Can you work these out from the model? Positions are in its coordinate system, mm. Face numbers are marked on the shaded views. A direction names the side the tool comes from. Give positions to 0.01 mm unless a question says otherwise; leave off trailing zeros. Loops run counter-clockwise (first coordinate to the right, second up) from the corner with the lowest first, then second, coordinate; pieces in that order, holes last. Notation, with made-up numbers: (80, 43) -> (86, 43) arc R25 ccw to (86, 60) -> close; hole circle Ø7 at (-19, 66). An arc over 180 degrees is marked (long way). One line per question, with ' | ' between items.
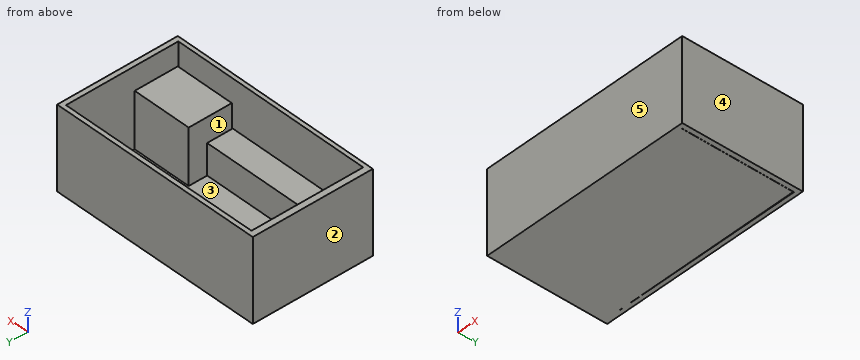
from build123d import *

# Parameters (mm, degrees)
F1_DEPTH = 76.708
F2_W     = 133.829683
F2_H     = 23.887876
F3_DEPTH = 32.512
F4_W     = 55.258706
F4_H     = 40.292808
F5_DEPTH = 55.372
F6_W     = 189.376198
F6_H     = 104.761295
F7_DEPTH = 3.81
F8_W     = 187.649362
F8_H     = 20.434209
F9_DEPTH = 35.306


with BuildPart() as f1:
    # F0 (on Top) → F1 (new body)
    with BuildSketch(Plane.XY):
        Polygon((99.436894, 56.841634), (-100.300305, 56.266025), (-100.300305, -55.97822), (99.436894, -55.97822), align=None)
        Polygon((-94.544195, -52.236743), (-94.544195, 52.236743), (94.832003, 52.81236), (94.832003, -52.236743), align=None, mode=Mode.SUBTRACT)
    extrude(amount=F1_DEPTH)

    # F2 (on Top) → F3 (join)
    with BuildSketch(Plane.XY):
        with Locations((-27.773253, -40.292805)):
            Rectangle(F2_W, F2_H)
    extrude(amount=F3_DEPTH)

    # F4 (on Top) → F5 (join)
    with BuildSketch(Plane.XY):
        with Locations((66.770941, -31.226925)):
            Rectangle(F4_W, F4_H)
    extrude(amount=F5_DEPTH)

    # F6 (on Top) → F7 (join)
    with BuildSketch(Plane.XY):
        with Locations((4e-06, -0.143905)):
            Rectangle(F6_W, F6_H)
    extrude(amount=F7_DEPTH)

    # F8 (on Top) → F9 (join)
    with BuildSketch(Plane.XY):
        with Locations((4e-06, 40.868416)):
            Rectangle(F8_W, F8_H)
    extrude(amount=F9_DEPTH)


solid = f1.part
Q1. For pin 1 Ø5 at (x, z) = (11.5, 43) entering from +Y; pin 2 Ø16.5 at (x, y) = (-46, 44.5) entering from +Z; pin 3 Ø25 at (x, z) = (41.5, 15.5) entering from +Y; pin 4 Ø20 at (x, y) = (64, -24) entering from +Z, each with a flat end and sliding along its axis, tell me the tip position at first contact or that it passes through.
Entries:
pin 1: y = 56.6 | pin 2: z = 76.71 | pin 3: y = 56.71 | pin 4: z = 55.37
Q2. If we section it at B-B (y = -48): Write out the boundary of the cut face in (x, z).
Entries:
outline: (-100.3, 0) -> (94.69, 0) -> (94.69, 3.81) -> (94.4, 3.81) -> (94.4, 55.37) -> (39.14, 55.37) -> (39.14, 32.51) -> (-94.54, 32.51) -> (-94.54, 76.71) -> (-100.3, 76.71) -> close; (94.83, 0) -> (99.44, 0) -> (99.44, 76.71) -> (94.83, 76.71) -> close
Q3. On a 3-axis mill with a long thin cutter (end or side, diameter ignored), from which of +Z, -Z, +X, -X, +Y, -Y can I reach the whole of each face in a straight line? I mean the marked faces 1 and 2. Say none if no direction works.
Entries:
face 1: +Z | face 2: +Z, -Z, -X, +Y, -Y
Q4. If I drill on probe 1 along X at (y, z) = (-35.5, 53); probe 2 along Y at (x, z) = (90.5, 9); probe 3 along X at (y, z) = (32.5, 15), over which ranges is the centre line in solid material (lowest first)? Write a range as from..to.
Entries:
probe 1: -100.3..-94.54, 39.14..94.4, 94.83..99.44 | probe 2: -55.98..-52.24, -51.37..-11.08, 30.65..51.09, 52.8..56.82 | probe 3: -100.3..-94.54, -93.82..93.82, 94.83..99.44
Q5. If we mould it in two halves opening along X, with no side actions, what happens to the marked faces 3, 4 and 5? For each: pulls with the +X half, pulls with the -X half, needs draft (parallel to the pull), parting line crosses it, or undercut.
Entries:
face 3: undercut | face 4: pulls with the +X half | face 5: needs draft
Q6. If we section it at A-A (z = 11.5): Write out the boundary of the cut face in (x, y), plus the area to 3 significant figures.
Entries:
outline: (-100.3, -55.98) -> (99.44, -55.98) -> (99.44, 56.84) -> (-100.3, 56.27) -> close; (-93.82, 30.65) -> (93.82, 30.65) -> (93.82, 51.09) -> (-93.82, 51.09) -> close; hole (-94.54, -28.35) -> (39.14, -28.35) -> (39.14, -11.08) -> (94.4, -11.08) -> (94.4, -51.37) -> (39.14, -51.37) -> (39.14, -52.24) -> (94.83, -52.24) -> (94.83, 52.81) -> (-94.54, 52.24) -> close | area: 11,900 mm²
Q7. If we section it at D-D (y = 37): Write out the boundary of the cut face in (x, z), plus the area to 3 significant figures.
Entries:
outline: (-100.3, 0) -> (94.69, 0) -> (94.69, 3.81) -> (93.82, 3.81) -> (93.82, 35.31) -> (-93.82, 35.31) -> (-93.82, 3.81) -> (-94.54, 3.81) -> (-94.54, 76.71) -> (-100.3, 76.71) -> close; (94.83, 0) -> (99.44, 0) -> (99.44, 76.71) -> (94.83, 76.71) -> close | area: 7,430 mm²
Q8. If we section it at C-C (x = 14.5): Write out the boundary of the cut face in (y, z), plus the area to 3 significant figures.
Entries:
outline: (-55.98, 0) -> (52.24, 0) -> (52.24, 3.81) -> (51.09, 3.81) -> (51.09, 35.31) -> (30.65, 35.31) -> (30.65, 3.81) -> (-28.35, 3.81) -> (-28.35, 32.51) -> (-52.24, 32.51) -> (-52.24, 76.71) -> (-55.98, 76.71) -> close; (52.57, 0) -> (56.6, 0) -> (56.6, 76.71) -> (52.57, 76.71) -> close | area: 2,320 mm²
